Verification items for the finished model (mm, model axes). A direction names the side the tool comes from. Coordinates: 2 decimals unless noted, no trailing zeros. Write each loop counter-clockwise with the first axis right and the second up, starting at its lowest first coordinate (ties: lowest second). Pieces come first, ordered by that corner, then holes. Notation, with made-up numbers: (64, 64.25) -> (85, 64.25) arc R32 ccw to (85, 103.25) -> close; hole circle Ø5 at (79.25, -34.75). An arc over 180 degrees is marked (long way). Answer in a Markdown table with one row per item.
Autodesk Inventor part; units mm, degrees
ref_plane "YZ Plane" through (0, 0, 0) normal (1, 0, 0) x (0, 1, 0)
ref_plane "XZ Plane" through (0, 0, 0) normal (0, 1, 0) x (-1, 0, 0)
ref_plane "XY Plane" through (0, 0, 0) normal (0, 0, 1) x (1, 0, 0)
ref_plane "作業平面1" through (0, 8, 0) normal (0, 1, 0) x (1, 0, 0)
sketch "スケッチ2" plane through (0, 8, 0) normal (0, 1, 0) x (1, 0, 0)
  arc A0 (28.3537, 29.9285) -> (28.3537, 54.5732) centre (-4.0051, 42.2508) ccw
  arc A1 (39.0644, 29.9285) -> (63.709, 29.9285) centre (51.3867, 62.2873) ccw
  line L0 (28.3537, 29.9285) -> (39.0644, 29.9285)
  arc A2 (39.0644, 19.2178) -> (39.0644, -5.4268) centre (71.4231, 6.8955) ccw
  line L1 (39.0644, 29.9285) -> (39.0644, 19.2178)
  arc A3 (28.3537, -5.4268) -> (28.3537, 19.2178) centre (-4.0051, 6.8955) ccw
  line L2 (39.0644, 19.2178) -> (28.3537, 19.2178)
  line L3 (28.3537, 19.2178) -> (28.3537, 29.9285)
  arc A4 (3.709, 29.9285) -> (28.3537, 29.9285) centre (16.0314, 62.2873) ccw
  line L4 (39.0644, 29.9285) -> (28.3537, 19.2178)
  line L5 (28.3537, 29.9285) -> (39.0644, 19.2178)
  circle A5 centre (33.709, 24.5732) radius 3
  circle A6 centre (33.709, 24.5732) radius 89.9592
  circle A7 centre (33.709, 24.5732) radius 15
  circle A8 centre (33.709, 24.5732) radius 12
  line L6 (30.4879, 39.2232) -> (30.052, 36.0024)
  line L7 (19.059, 27.7943) -> (22.2798, 28.2302)
  line L8 (30.4879, 9.9231) -> (30.052, 13.144)
  circle A9 centre (33.709, 24.5732) radius 15
  circle A10 centre (33.709, 24.5732) radius 12
  line L9 (19.059, 21.352) -> (22.2798, 20.9162)
  line L10 (48.3591, 21.352) -> (45.1382, 20.9162)
  circle A11 centre (33.709, 24.5732) radius 15
  circle A12 centre (33.709, 24.5732) radius 12
  line L11 (36.9302, 9.9231) -> (37.366, 13.144)
  line L12 (36.9302, 39.2232) -> (37.366, 36.0024)
  circle A13 centre (33.709, 24.5732) radius 15
  circle A14 centre (33.709, 24.5732) radius 12
  line L13 (48.3591, 27.7943) -> (45.1382, 28.2302)
  point P0 (0, 0)
  point P1 (22.2798, 28.2302)
  point P2 (30.052, 36.0024)
  point P3 (30.4879, 39.2232)
  point P4 (19.059, 27.7943)
  point P5 (30.4879, 9.9231)
  point P6 (30.052, 13.144)
  point P7 (37.366, 13.144)
  point P8 (36.9302, 9.9231)
  point P9 (45.1382, 28.2302)
  point P10 (48.3591, 27.7943)
  dimension "d6" = 6
  dimension "d7" = 30
  dimension "d8" = 24
  dimension "d13" = 360
extrude "押し出し2" add sketch "スケッチ2" along normal blind 8.5 contours L6 A0 | A8 L7 A7 L6 | A4 L7 | L12 A7 L13 A8 | L8 A7 L9 A8 | A8 L10 A7 L11
ref_plane "作業平面2" through (0, 16.5, 0) normal (0, 1, 0) x (1, 0, 0)
sketch "スケッチ4" plane through (0, 16.5, 0) normal (0, 1, 0) x (1, 0, 0)
  arc A0 (30.052, 36.0024) -> (22.2798, 28.2302) centre (33.709, 24.5732) ccw
  arc A1 (28.3537, 29.9285) -> (30.052, 36.0024) centre (-4.0051, 42.2508) ccw
  line L0 (22.2798, 28.2302) -> (30.052, 36.0024)
  line L1 (30.052, 36.0024) -> (26.1659, 32.1163)
  arc A2 (37.366, 13.144) -> (45.1382, 20.9162) centre (33.709, 24.5732) ccw
  line L2 (33.709, 24.5732) -> (26.1659, 32.1163)
  circle A3 centre (33.709, 24.5732) radius 15
  point P0 (0, 0)
extrude "押し出し3" add sketch "スケッチ4" along normal blind 10 contours L0 A0 | A1 L2 L0 | A3
sketch "スケッチ6" plane through (33.709, 26.5, -24.5732) normal (0, 1, 0) x (1, 0, 0)
  circle A0 centre (0, 0) radius 15
  circle A1 centre (0, 0) radius 12
  arc A2 (-12.6369, -8.0814) -> (-10.6675, -5.4958) centre (-39.1679, 14.1679) ccw
  line L0 (-12.6369, -8.0814) -> (-10.6675, -5.4958)
  line L1 (-5.4958, -10.6675) -> (-8.0814, -12.6369)
  arc A3 (8.0814, -12.6369) -> (5.4958, -10.6675) centre (-14.1679, -39.1679) ccw
  line L2 (10.6675, -5.4958) -> (12.6369, -8.0814)
  arc A4 (12.6369, 8.0814) -> (10.6675, 5.4958) centre (39.1679, -14.1679) ccw
  line L3 (5.4958, 10.6675) -> (8.0814, 12.6369)
  arc A5 (-8.0814, 12.6369) -> (-5.4958, 10.6675) centre (14.1679, 39.1679) ccw
  line L4 (-10.6675, 5.4958) -> (-12.6369, 8.0814)
  point P0 (-33.709, -24.5732)
  point P1 (-10.6675, 5.4958)
  point P2 (-12.6369, 8.0814)
  point P3 (-12.6369, -8.0814)
  point P4 (-10.6675, -5.4958)
  point P5 (8.0814, -12.6369)
  point P6 (5.4958, -10.6675)
  point P7 (-5.4958, -10.6675)
  point P8 (-8.0814, -12.6369)
  point P9 (12.6369, 8.0814)
  point P10 (10.6675, 5.4958)
  point P11 (-8.0814, 12.6369)
  point P12 (-5.4958, 10.6675)
  point P13 (5.4958, 10.6675)
  dimension "d19" = 24
  dimension "d20" = 30
  dimension "d23" = 360
extrude "押し出し4" add sketch "スケッチ6" along normal blind 8.5 contours A0 L2 A1 A4 | L3 A1 A5 A0 | A0 L1 A1 A3 | L4 A1 L0 A0
sketch "スケッチ7" plane through (0, 16.5, 0) normal (0, -1, 0) x (1, 0, 0)
  arc A0 (44.3766, -30.0689) -> (44.3766, -19.0774) centre (33.709, -24.5732) ccw
  line L0 (33.709, -24.5732) -> (48.7, -24.5732)
  circle A1 centre (33.709, -24.5732) radius 3
  point P0 (0, 0)
  dimension "d27" = 6
extrude "押し出し5" cut sketch "スケッチ7" against normal blind 10
properties part number "隙間パーツ"
1. Go/stop test with flat-tipped pins: pin 1 (9.5 mm diameter, centred on x = 33.71, z = -24.57, fed in from +Y); pin 2 (1.5 mm diameter, centred on y = 30, z = -17.5, fed in from +X); pin 3 (5 mm diameter, centred on y = 23, z = -14.5, fed in from -X); pin 4 (12 mm diameter, centred on x = 32, z = -14.5, fed in from +Y). Record where each tip stops, or that it passes through.
Findings below:
| item | result |
|---|---|
| pin 1 | stops at y = 26.5 |
| pin 2 | stops at x = 47.31 |
| pin 3 | stops at x = 20.76 |
| pin 4 | stops at y = 35 |
2. Sectioned sample at C-C, the plane z = -23. Record the cut outline in (x, y), and give its area (3 significant figures).
Findings below:
| item | result |
|---|---|
| outline | (18.79, 16.5) -> (31.15, 16.5) -> (31.15, 26.5) -> (21.81, 26.5) -> (21.81, 35) -> (18.79, 35) -> close; (36.26, 16.5) -> (48.63, 16.5) -> (48.63, 35) -> (45.61, 35) -> (45.61, 26.5) -> (36.26, 26.5) -> close |
| area | 299 mm² |
3. Sectioned sample at B-B, the plane x = 34.75. Record the cut outline in (y, z), and give its area (3 significant figures).
Findings below:
| item | result |
|---|---|
| outline | (16.5, -39.54) -> (35, -39.54) -> (35, -36.53) -> (26.5, -36.53) -> (26.5, -27.39) -> (16.5, -27.39) -> close; (16.5, -21.76) -> (26.5, -21.76) -> (26.5, -12.62) -> (35, -12.62) -> (35, -9.61) -> (16.5, -9.61) -> close |
| area | 294 mm² |
4. Release check for a two-part mould opening along X. For faces 6 (the face through (22.043, 30.69, -17.767)), 7 (the face through (26.938, 30.69, -12.935)), 8 (the face through (47, 35, -25)) record: released by +X, released by -X, zero draft, split by the parting line, or undercut.
Findings below:
| item | result |
|---|---|
| face 6 | undercut |
| face 7 | released by -X |
| face 8 | zero draft |
5. Sectioned sample at D-D, the plane z = -15.5. Record the cut outline in (x, y).
Findings below:
| item | result |
|---|---|
| outline | (21.76, 8) -> (25.86, 8) -> (25.86, 16.5) -> (41.56, 16.5) -> (41.56, 8) -> (45.65, 8) -> (45.65, 26.5) -> (21.76, 26.5) -> close |
6. Access from +Z, -Z, +X, -X, +Y, -Y to the whole of each face (thin tool, end or side, straight path). Record for faces 1 (the face through (40.48, 30.69, -36.21)), 2 (the face through (22.071, 30.69, -31.344)), 3 (the face through (37.145, 12.19, -11.511)), 4 (the face through (45.71, 30.69, -24.65)), 5 (the face through (25, 8, -16)).
Findings below:
| item | result |
|---|---|
| face 1 | +X, +Y |
| face 2 | -Z, +Y |
| face 3 | -Y |
| face 4 | +Y |
| face 5 | +Z, -Z, +X, -X, -Y |
7. Sectioned sample at A-A, the plane y = 32. Record the cut outline in (x, z), and give its area (3 significant figures).
Findings below:
| item | result |
|---|---|
| outline | (21.07, -32.65) -> (23.04, -30.07) arc R12 cw to (23.04, -19.08) -> (21.07, -16.49) arc R15 ccw to start; (25.63, -37.21) arc R15 ccw to (41.79, -37.21) -> (39.2, -35.24) arc R12 cw to (28.21, -35.24) arc R34.68 ccw to start; (25.63, -11.94) -> (28.21, -13.91) arc R12 cw to (39.2, -13.91) arc R34.68 ccw to (41.79, -11.94) arc R15 ccw to start; (44.38, -30.07) arc R34.68 ccw to (46.35, -32.65) arc R15 ccw to (46.35, -16.49) -> (44.38, -19.08) arc R12 cw to start |
| area | 171 mm² |
8. Material ranges on probe 1 along X at (y, z) = (29.25, -24.5); probe 2 along Y at (x, z) = (25.25, -22.5); probe 3 along Y at (x, z) = (30.25, -12), recorded low to high. Write a range as from..to.
Findings below:
| item | result |
|---|---|
| probe 1 | x = 18.71..21.71, 45.71..48.71 |
| probe 2 | y = 16.5..26.5 |
| probe 3 | y = 16.5..35 |
